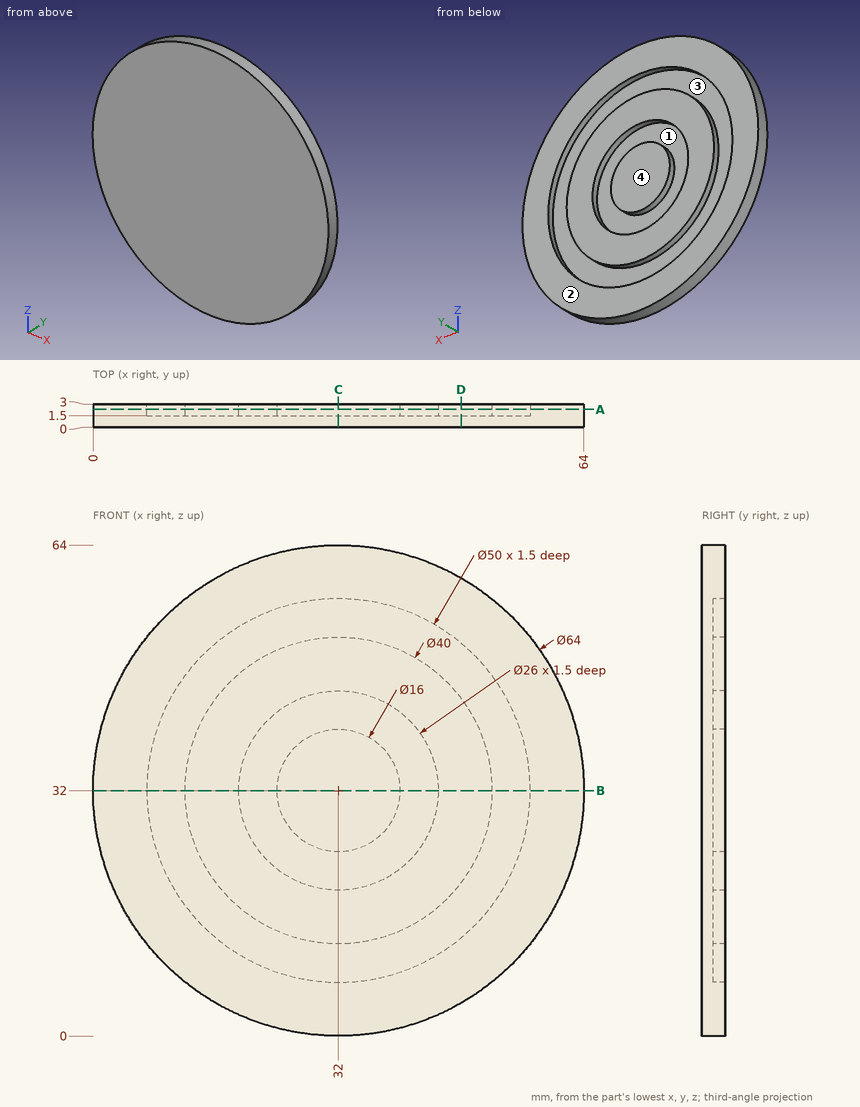
Geometry: see drawing. Coordinates: mm, zero at the bounding-box minimum. A direction names the side the tool comes from. Coordinates: 2 decimals unless noted, no trailing zeros. Write each loop counter-clockwise with the first axis right and the second up, starting at its lowest first coordinate (ties: lowest second). Pieces come first, ordered by that corner, then holes. Notation, with made-up numbers: M -15,30.5 L -8,30.5 A7 cw -8,42.5 Z; hole C 21.5,76 d1. An arc over 180 degrees is marked long. Answer as a JSON object with one key per item and string values.
1. Cut plane A-A on y = 2.3. Output: boundary loops of the cut face in (x, z), plus the area to 3 significant figures.
Evaluation:
{"outline": "C 32,32 d64; C 32,32 d40; C 32,32 d16; hole C 32,32 d50; hole C 32,32 d26", "area": "2,180 mm^2"}
2. Contact query for flat-ended pins moving along their axis: P1, Ø1, axis at x = 47.5, y = 2, coming from the +Z side; P2, Ø12, axis at x = 45, z = 52.5, coming from the +Y side. Output: stop coordinate, or through.
Evaluation:
{"P1": "z = 60.27", "P2": "y = 3"}
3. Ray query, L1, parallel to Z at x = 32, y = 2.1; L2, parallel to Y at x = 33.5, z = 11; L3, parallel to X at y = 2.3, z = 36. Return the intervals inside material, ascending.
Evaluation:
{"L1": "0 to 7, 12 to 19, 24 to 40, 45 to 52, 57 to 64", "L2": "0 to 1.5", "L3": "0.25 to 7.32, 12.4 to 19.63, 25.07 to 38.93, 44.37 to 51.6, 56.68 to 63.75"}
4. Draft query along Z for the marked faces 3 and 4. Return one class per face: released by +Z, released by -Z, zero draft, split by the parting line, or undercut.
Evaluation:
{"face 3": "undercut", "face 4": "zero draft"}
5. Access query for the marked faces 1 and 2. Directions: +Z, -Z, +X, -X, +Y, -Y. A direction counts if a zero-diameter tool reaches every point of the face in a straight line with its end or side. Return the directions, or none.
Evaluation:
{"face 1": "+Y", "face 2": "+Z, -Z, +X, -X, +Y"}
6. Cut plane D-D on x = 48. Output: boundary loops of the cut face in (y, z), plus the area to 3 significant figures.
Evaluation:
{"outline": "M 0,4.29 L 3,4.29 L 3,12.79 L 1.5,12.79 L 1.5,20 L 3,20 L 3,44 L 1.5,44 L 1.5,51.21 L 3,51.21 L 3,59.71 L 0,59.71 Z", "area": "145 mm^2"}
7. Cut plane B-B on z = 32. Output: boundary loops of the cut face in (x, y), plus the area to 3 significant figures.
Evaluation:
{"outline": "M 0,0 L 64,0 L 64,3 L 57,3 L 57,1.5 L 52,1.5 L 52,3 L 45,3 L 45,1.5 L 40,1.5 L 40,3 L 24,3 L 24,1.5 L 19,1.5 L 19,3 L 12,3 L 12,1.5 L 7,1.5 L 7,3 L 0,3 Z", "area": "162 mm^2"}
8. Cut plane C-C on x = 32. Output: boundary loops of the cut face in (y, z), plus the area to 3 significant figures.
Evaluation:
{"outline": "M 0,0 L 3,0 L 3,7 L 1.5,7 L 1.5,12 L 3,12 L 3,19 L 1.5,19 L 1.5,24 L 3,24 L 3,40 L 1.5,40 L 1.5,45 L 3,45 L 3,52 L 1.5,52 L 1.5,57 L 3,57 L 3,64 L 0,64 Z", "area": "162 mm^2"}
